Verification items for the finished model (mm, model axes). Give positions to 0.01 mm unless a question says otherwise; leave off trailing zeros. Order: outer loops, then holes, each group sorted by start corner. A loop starts at its lowest first (then second) coordinate and runs counter-clockwise, first axis right, second up. Notation, with made-up numbers: (74.5, 76.25) -> (93.5, 76.25) arc R23 cw to (93.5, 84.25) -> close; hole circle Ø10 at (70, -18.75). An arc over 180 degrees is marked (long way). One line per question, with ' | ' between items. Start each with the question number.
Q1. Section check B-B on x = -3.25. Record the cut outline in (y, z).
Q2. Section check A-A on z = 30. Record the cut outline in (x, y).
Q3. Material ranges on probe 1 along Y at (x, z) = (-2.75, 143); probe 2 along X at (y, z) = (6.75, 110); probe 3 along X at (y, z) = (1.5, 113), recorded low to high. Write a range as [from, to].
Q4. Go/stop test with flat-tipped pins: pin 1 (2 mm diameter, centred on y = 5, z = 31.5, fed in from -X); pin 2 (4 mm diameter, centred on x = -0.5, y = 10.5, fed in from -Z); pin 3 (1.5 mm diameter, centred on x = 1, z = 26.5, fed in from +Y); pin 4 (2 mm diameter, centred on y = 2.5, z = 139, fed in from -X). Record where each tip stops, or that it passes through.
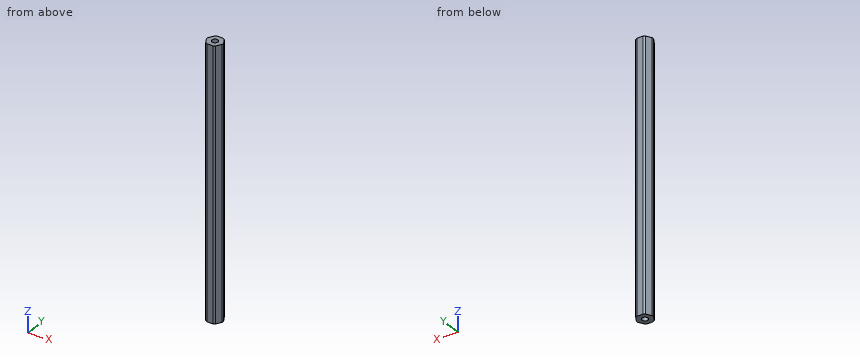
Autodesk Inventor part; units mm, degrees
ref_plane "YZ Plane" through (0, 0, 0) normal (1, 0, 0) x (0, 1, 0)
ref_plane "XZ Plane" through (0, 0, 0) normal (0, 1, 0) x (-1, 0, 0)
ref_plane "XY Plane" through (0, 0, 0) normal (0, 0, 1) x (1, 0, 0)
sketch "Sketch1" plane through (0, 0, 0) normal (0, 0, 1) x (1, 0, 0)
  circle A0 centre (-2.6438, 6.9447) radius 6.8758
  line L0 (-9.4616, 7.8359) -> (-6.8245, 12.4034)
  line L1 (-6.8245, 1.4859) -> (-9.4616, 6.0534)
  line L2 (-0.0068, 0.5947) -> (-5.2808, 0.5947)
  line L3 (4.174, 6.0534) -> (1.537, 1.4859)
  line L4 (1.537, 12.4034) -> (4.174, 7.8359)
  line L5 (-5.2808, 13.2947) -> (-0.0068, 13.2947)
  point P0 (0, 0)
  point P1 (1.537, 1.4859)
  dimension "d0" = 13.7516
  dimension "d4" = 360
extrude "Extrusion1" add sketch "Sketch1" along normal blind 228.6 contours A0 L3 L2 L1 L0 L5 L4
sketch "Sketch2" plane through (0, 0, 228.6) normal (0, 0, 1) x (1, 0, 0)
  circle A0 centre (-2.6438, 6.9447) radius 2.5527
  line L0 (-5.2808, 0.5947) -> (-0.0068, 0.5947)
  line L1 (-2.6438, 6.9447) -> (-5.2808, 0.5947) construction
  line L2 (-2.6438, 6.9447) -> (-0.0068, 0.5947) construction
  point P0 (0, 0)
  dimension "d8" = 5.1054
  dimension "d9" = 6.35
extrude "Extrusion2" cut sketch "Sketch2" against normal blind 228.6
equation "\"d6\" = d5"
equation "\"d10\" = d5"
equation "\"d5\" = 228.6"
properties part number "Thundershaft-7"
Filled in:
1) outline: (0.59, 0) -> (4.47, 0) -> (4.47, 228.6) -> (0.59, 228.6) -> close; (9.42, 0) -> (13.29, 0) -> (13.29, 228.6) -> (9.42, 228.6) -> close
2) outline: (-9.46, 6.05) -> (-6.82, 1.49) arc R6.88 ccw to (-5.28, 0.59) -> (-0.01, 0.59) arc R6.88 ccw to (1.54, 1.49) -> (4.17, 6.05) arc R6.88 ccw to (4.17, 7.84) -> (1.54, 12.4) arc R6.88 ccw to (-0.01, 13.29) -> (-5.28, 13.29) arc R6.88 ccw to (-6.82, 12.4) -> (-9.46, 7.84) arc R6.88 ccw to start; hole circle Ø5.11 at (-2.64, 6.94)
3) probe 1: [0.59, 4.39], [9.5, 13.29] | probe 2: [-9.52, -5.19], [-0.1, 4.23] | probe 3: [-6.83, 1.55]
4) pin 1: x = -9.43 | pin 2: z = 0 | pin 3: y = 13.18 | pin 4: x = -7.99
